Can you work these out from the model? Positions are in its coordinate system, mm. A direction names the side the tool comes from. Coordinates: 2 decimals unless noted, no trailing zeros. Loops run counter-clockwise (first coordinate to the right, second up) from the corner with the lowest first, then second, coordinate; pieces in that order, holes last.
```python
from build123d import *

# Parameters (mm, degrees)
RESSALTO_EXTRUS_O4_DEPTH = 20
ESBO_O8_W                = 6.5
ESBO_O8_H                = 6.5
CORTE_EXTRUS_O1_DEPTH    = 15
CORTE_EXTRUS_O2_START    = -1
CORTE_EXTRUS_O2_DEPTH    = 4
CHANFRO1_SIZE            = 0.2
CHANFRO2_SIZE            = 5
ESBO_O10_R               = 2.25
CORTE_EXTRUS_O3_DEPTH    = 214


with BuildPart() as part:
    # Esboço7 → Ressalto-extrusão4 (new body)
    with BuildSketch(Plane.XY):
        Polygon((0, 0), (100, 0), (100, 10), (70, 10), (55, 197), (45, 197), (30, 10), (0, 10), align=None)
    extrude(amount=RESSALTO_EXTRUS_O4_DEPTH)

    # Esboço8 → Corte-extrusão1 (cut)
    with BuildSketch(Plane(origin=(0, 197, 0), x_dir=(1, 0, 0), z_dir=(0, 1, 0))):
        with Locations((50, -10)):
            Rectangle(ESBO_O8_W, ESBO_O8_H)
    extrude(amount=-CORTE_EXTRUS_O1_DEPTH, mode=Mode.SUBTRACT)

    # Esboço9 → Corte-extrusão2 (cut)
    with BuildSketch(Plane(origin=(0, 197, 0), x_dir=(1, 0, 0), z_dir=(0, 1, 0)).offset(CORTE_EXTRUS_O2_START)):
        with BuildLine():
            Line((48.75, -6.75), (51.25, -6.75))
            ThreePointArc((51.25, -6.75), (50, -6.079156198), (48.75, -6.75))
        make_face()
        with BuildLine():
            Line((53.25, -8.75), (53.25, -11.25))
            ThreePointArc((53.25, -11.25), (53.920843802, -10), (53.25, -8.75))
        make_face()
        with BuildLine():
            Line((46.75, -8.75), (46.75, -11.25))
            ThreePointArc((46.75, -11.25), (46.079156198, -10), (46.75, -8.75))
        make_face()
        with BuildLine():
            Line((48.75, -13.25), (51.25, -13.25))
            ThreePointArc((51.25, -13.25), (50, -13.920843802), (48.75, -13.25))
        make_face()
    extrude(amount=-CORTE_EXTRUS_O2_DEPTH, mode=Mode.SUBTRACT)

    # Chanfro1
    chanfro1_edges = [part.edges().sort_by_distance(p)[0] for p in [
        (50, 196, 6.75),
        (53.25, 196, 10),
        (50, 196, 13.25),
        (46.75, 196, 10),
    ]]
    chamfer(chanfro1_edges, length=CHANFRO1_SIZE)

    # Chanfro2
    chanfro2_edges = [part.edges().sort_by_distance(p)[0] for p in [
        (50, 197, 20),
        (50, 197, 0),
    ]]
    chamfer(chanfro2_edges, length=CHANFRO2_SIZE)

    # Esboço10 → Corte-extrusão3 (cut, through all)
    with BuildSketch(Plane(origin=(0, 10, 0), x_dir=(1, 0, 0), z_dir=(0, 1, 0))):
        with Locations(Location((15, -10, 0), (0, 0, 180))):
            Circle(ESBO_O10_R)
        with Locations(Location((85, -10, 0), (0, 0, 180))):
            Circle(ESBO_O10_R)
    extrude(amount=-CORTE_EXTRUS_O3_DEPTH, mode=Mode.SUBTRACT)


solid = part.part
```
Item 1: Suppose I cut it at A-A, the plane x = 15. Please give me the cut outline in (y, z).
Results are:
outline: (0, 0) - (10, 0) - (10, 7.75) - (0, 7.75) - close; (0, 12.25) - (10, 12.25) - (10, 20) - (0, 20) - close
Item 2: I'm going to push flat-ended pins straight in: P1, Ø1.5, axis at y = 86, z = 7, coming from the -X side; P2, Ø1.5, axis at x = 88.5, z = 5.5, coming from the +Y side; P3, Ø2, axis at y = 188, z = 9, coming from the +X side. Where does each tip first touch, or does it pass through?
Results are:
P1: stops at x = 36.04
P2: stops at y = 10
P3: stops at x = 55.8
Item 3: We'd pull the mould along Z, two halves only. Please class faces 4 (the face through (53.25, 190, 10)), 5 (the face through (82.854, 5.07, 10.676)), 6 (the face through (50, 75, 0)), 7 (the face through (15.2, 10, 7.6)): +Z half, -Z half, draft (parallel to the pull), parting line (faces both ways), or undercut.
Results are:
face 4: undercut
face 5: undercut
face 6: -Z half
face 7: draft
Item 4: I need wall thicknesses on line 1 along Z through (x, y) = (15, 5); line 2 along Y through (x, z) = (20, 11.75); line 3 along Y through (x, z) = (47, 2.75). Which ranges of each line are inside material? Lowest first, please.
Results are:
line 1: z = 0 to 7.75, 12.25 to 20
line 2: y = 0 to 10
line 3: y = 0 to 194.75
Item 5: On a 3-axis mill with a long thin cutter (end or side, diameter ignored), from which of +Z, -Z, +X, -X, +Y, -Y can I reach the whole of each face in a straight line? I mean faces 1 (the face through (50, 190, 13.25)), 2 (the face through (85.2, 10, 7.6)), 3 (the face through (50, 194, 18)). Say none if no direction works.
Results are:
face 1: +Y
face 2: +Z, -Z, +X, +Y
face 3: +Z, +X, -X, +Y
Item 6: Suppose I cut it at C-C, the plane y = 83. Please give me the cut outline in (x, z).
Results are:
outline: (35.86, 0) - (64.14, 0) - (64.14, 20) - (35.86, 20) - close
Item 7: Suppose I cut it at D-D, the plane x = 78.5. Please give me the cut outline in (y, z).
Results are:
outline: (0, 0) - (10, 0) - (10, 20) - (0, 20) - close
Item 8: Suppose I cut it at B-B, the plane z = 2.5. Please give me the cut outline in (x, y), plus the area to 3 significant figures.
Results are:
outline: (0, 0) - (100, 0) - (100, 10) - (70, 10) - (55.2, 194.5) - (44.8, 194.5) - (30, 10) - (0, 10) - close
area: 5,650 mm2
